Read the model definition and answer for the solid it produces. Units are mm, in the model's axes. A direction names the side the tool comes from. Give positions to 0.01 mm unless a question says otherwise; leave off trailing zeros. Loops run counter-clockwise (first coordinate to the right, second up) from the corner with the lowest first, then second, coordinate; pieces in that order, holes last. Notation, with made-up numbers: (-23, 78) - (24, 78) arc R15 cw to (24, 88) - close; hole circle Ø3 at (57, 44). An arc over 180 degrees is marked (long way). Put each result on its own line as item: value. Start each with the question number.
1. A cutting plane is placed at B-B, the plane y = 98. Determine the outline of the cut face in (x, z).
2. Given pin 1 Ø2 at (y, z) = (43.5, 3.5) entering from +X; pin 2 Ø4 at (x, y) = (-6, 90) entering from +Z; pin 3 Ø8 at (x, y) = (20.5, 104.5) entering from -Z; pin 4 Ø2 at (y, z) = (61, 3.5) entering from -X, each flat-ended and moving along its own axis, determine where each tip first touches the part or whether it passes through.
3. Consider L1, parallel to Y at x = -1.5, z = -13; L2, parallel to Y at x = -6.5, z = -5.5; L3, parallel to X at y = 81, z = -1. Determine where each line is inside the solid, lowest interval first. Write a range as from..to.
4. A cutting plane is placed at A-A, the plane y = 30. Determine the outline of the cut face in (x, z).
5. For a pull along Y with two mould halves and no side action, classify faces 4 (the flat face through (-2.4, -8, 2.1)), 5 (the flat face through (0, 134, 0)), 6 (the cylindrical face through (-15.821, 119.367, -20.633)) as released by +Y, released by -Y, zero draft, split by the parting line, or undercut.
6. For faces 1 (the cylindrical face through (-15.821, 49.37, -20.633)), 2 (the flat face through (5, 0, 9)), 3 (the cylindrical face through (0.33, 104.93, -7.493)), determine the directions among +Z, -Z, +X, -X, +Y, -Y from which every point of the face is accessible in a straight line to the end or side of a thin tool.
```python
from build123d import *

# Parameters (mm, degrees)
SKETCH1_R           = 26
BOSS_EXTRUDE2_DEPTH = 100
SKETCH2_R           = 7.5
BOSS_EXTRUDE4_DEPTH = 10
SKETCH3_R           = 26
BOSS_EXTRUDE5_DEPTH = 24
FILLET1_R           = 5
FILLET2_R           = 5
FILLET3_R           = 5
SKETCH4_R           = 10
BOSS_EXTRUDE6_DEPTH = 8
SKETCH5_R           = 2.935336569
BOSS_EXTRUDE7_DEPTH = 4
SKETCH6_R           = 6.699984979
BOSS_EXTRUDE8_DEPTH = 40
SKETCH7_R           = 1
BOSS_EXTRUDE9_DEPTH = 30


with BuildPart() as part:
    # Sketch1 → Boss-Extrude2 (new body)
    with BuildSketch(Plane(origin=(0, 0, 0), x_dir=(1, 0, 0), z_dir=(0, 1, 0))):
        with Locations(Location((0, 0, 0), (0, 0, 270))):
            Circle(SKETCH1_R)
    extrude(amount=BOSS_EXTRUDE2_DEPTH)

    # Sketch2 → Boss-Extrude4 (add)
    with BuildSketch(Plane(origin=(0, 100, 0), x_dir=(1, 0, 0), z_dir=(0, 1, 0))):
        with Locations(Location((0, 0, 0), (0, 0, 270))):
            Circle(SKETCH2_R)
    extrude(amount=BOSS_EXTRUDE4_DEPTH)

    # Sketch3 → Boss-Extrude5 (add)
    with BuildSketch(Plane(origin=(0, 110, 0), x_dir=(1, 0, 0), z_dir=(0, 1, 0))):
        with Locations(Location((0, 0, 0), (0, 0, 270))):
            Circle(SKETCH3_R)
    extrude(amount=BOSS_EXTRUDE5_DEPTH)

    # Fillet1
    fillet1_edges = [part.edges().sort_by_distance(p)[0] for p in [
        (0, 0, -26),
    ]]
    fillet(fillet1_edges, radius=FILLET1_R)

    # Fillet2
    fillet2_edges = [part.edges().sort_by_distance(p)[0] for p in [
        (0, 100, -26),
    ]]
    fillet(fillet2_edges, radius=FILLET2_R)

    # Fillet3
    fillet3_edges = [part.edges().sort_by_distance(p)[0] for p in [
        (0, 134, -26),
    ]]
    fillet(fillet3_edges, radius=FILLET3_R)

    # Sketch4 → Boss-Extrude6 (add)
    with BuildSketch(Plane.XZ):
        with Locations(Location((0, 0, 0), (0, 0, 90))):
            Circle(SKETCH4_R)
    extrude(amount=BOSS_EXTRUDE6_DEPTH)

    # Sketch5 → Boss-Extrude7 (add)
    with BuildSketch(Plane.XZ.offset(8)):
        with Locations(Location((0, 0, 0), (0, 0, 270))):
            Circle(SKETCH5_R)
    extrude(amount=BOSS_EXTRUDE7_DEPTH)

    # Sketch6 → Boss-Extrude8 (add)
    with BuildSketch(Plane.XZ.offset(12)):
        with Locations(Location((0, 0, 0), (0, 0, 270))):
            Circle(SKETCH6_R)
    extrude(amount=BOSS_EXTRUDE8_DEPTH)

    # Sketch7 → Boss-Extrude9 (add)
    with BuildSketch(Plane.XZ.offset(52)):
        with Locations(Location((0, 0, 0), (0, 0, 270))):
            Circle(SKETCH7_R)
    extrude(amount=BOSS_EXTRUDE9_DEPTH)


solid = part.part
```
Return value:
1. outline: circle Ø50 at (0, 0)
2. pin 1: stops at x = 25.88
2. pin 2: stops at z = 25.69
2. pin 3: passes through
2. pin 4: stops at x = -25.88
3. L1: y = 0..100, 110..134
3. L2: y = -8..100, 110..134
3. L3: x = -25.98..25.98
4. outline: circle Ø52 at (0, 0)
5. face 4: undercut
5. face 5: released by +Y
5. face 6: zero draft
6. face 1: +Y, -Y
6. face 2: -Y
6. face 3: none
